Autodesk Inventor part; units mm, degrees
ref_plane "Work Plane1" through (0, -4, 9.6) normal (1, 0, 0) x (0, 0, -1)
ref_plane "YZ Plane" through (0, 0, 0) normal (1, 0, 0) x (0, 1, 0)
ref_plane "XZ Plane" through (0, 0, 0) normal (0, 1, 0) x (-1, 0, 0)
sketch "Sketch1" plane through (0, 0, 0) normal (0, 0, 1) x (1, 0, 0)
  line L0 (-4, -4) -> (4, -4)
  line L1 (4, -4) -> (4, 4)
  line L2 (4, 4) -> (-4, 4)
  line L3 (-4, 4) -> (-4, -4)
  line L4 (-4, -4) -> (4, 4) construction
  line L5 (4, -4) -> (-4, 4) construction
  circle A0 centre (0, 0) radius 2.4
  dimension "d0" = 8
  dimension "d1" = 8
  dimension "d2" = 4.8
extrude "Extrusion1" add sketch "Sketch1" along normal blind 9.6 contours L3 L2 L1 L0 | A0
extrude "Extrusion2" add sketch "Sketch1" along normal blind 11.3 contours A0
extrude "Extrusion3" cut sketch "Sketch1" along normal blind 1.7 contours A0
pattern_linear "Rectangular Pattern1" count 10 spacing 8 along (0, 1, 0) of "Extrusion1", "Extrusion2", "Extrusion3"
sketch "Sketch2" plane through (4, -4, 9.6) normal (1, 0, 0) x (0, 0, -1)
  circle A0 centre (4, 8) radius 2.4
  circle A1 centre (4, 8) radius 3.1
  line L0 (9.6, 0) -> (9.6, 80)
  line L1 (9.6, 0) -> (0, 0)
  point P0 (9.6, 4)
  dimension "d12" = 4.8
  dimension "d14" = 6.2
  dimension "d22" = 8
  dimension "d23" = 5.6
ref_plane "Work Plane1" through (0, -4, 9.6) normal (1, 0, 0) x (0, 0, -1)
extrude "Extrusion4" cut sketch "Sketch2" against normal up to next contours A0
extrude "Extrusion5" cut sketch "Sketch2" against normal blind 0.8
mirror "Mirror1" about plane through (0, -4, 9.6) normal (1, 0, 0) of "Extrusion5"
pattern_linear "Rectangular Pattern2" count 9 spacing 8 along (0, 1, 0) of "Extrusion4", "Extrusion5", "Mirror1"
equation "\"d11\" = d0"
equation "\"d21\" = d0"
properties part number "LEGO Technic Brick 1x10 with Holes"
CAD build for the part. Positions are in the model's coordinates, mm. A direction names the side the tool comes from. Round coordinates to 2 decimals unless told otherwise and drop trailing zeros. Loops run counter-clockwise (first coordinate to the right, second up) from the corner with the lowest first, then second, coordinate; pieces in that order, holes last. Notation, with made-up numbers: (4.5, -27.75) - (35.5, -27.75) arc R13 cw to (35.5, -8.75) - close; hole circle Ø9 at (45.5, -21). An arc over 180 degrees is marked (long way). Put each result on its own line as item: value.
1. Slice it at C-C on z = 6.25. Give the number of separate pieces and of enclosed holes in the cut face, and give its area (3 significant figures).
Geometry check:
separate pieces: 10
enclosed holes: 0
area: 287 mm²
2. Pin check, flat tips, straight feed: P1, Ø4, axis at x = -1, y = 16.5, coming from the -Z side; P2, Ø1, axis at x = 0, y = 47, coming from the -Z side. Stop position of each tip, or through.
Geometry check:
P1: z = 0
P2: z = 1.7
3. Wall check: line 1 (Z direction, x = 2.25, y = 47); line 2 (X direction, y = 23, z = 5.5); line 3 (Z direction, x = 3.25, y = 3.5). Give the ranges that are in metal, low to high.
Geometry check:
line 1: 0 to 9.6
line 2: -3.2 to 3.2
line 3: 0 to 2.54, 8.66 to 9.6
4. Two-plate mould, pull along Z, no slides. Class faces 6 (the cylindrical face through (-3.606, 13.187, 2.736)), 7 (the cylindrical face through (-0.31, 61.62, 10.44)), 8 (the flat face through (0, 8, 11.3)): released by +Z, released by -Z, zero draft, split by the parting line, or undercut.
Geometry check:
face 6: undercut
face 7: zero draft
face 8: released by +Z
5. Slice it at A-A on y = 28. List the corners of the cut face in (x, z).
Geometry check:
outline: (-4, 0) - (4, 0) - (4, 2.5) - (3.2, 2.5) - (3.2, 3.2) - (-3.2, 3.2) - (-3.2, 2.5) - (-4, 2.5) - close; (-4, 8.7) - (-3.2, 8.7) - (-3.2, 8) - (3.2, 8) - (3.2, 8.7) - (4, 8.7) - (4, 9.6) - (-4, 9.6) - close
6. Slice it at B-B on y = 40. List the corners of the cut face in (x, z).
Geometry check:
outline: (-4, 0) - (-2.4, 0) - (-2.4, 1.7) - (2.4, 1.7) - (2.4, 0) - (4, 0) - (4, 9.6) - (2.4, 9.6) - (2.4, 11.3) - (-2.4, 11.3) - (-2.4, 9.6) - (-4, 9.6) - close
7. 3-axis set-ups, long thin cutter, end or side, ignore diameter. For faces 1 (the cylindrical face through (1.29, 13.976, 10.438)), 2 (the cylindrical face through (0.045, 62.024, 4.31)), 3 (the cylindrical face through (-3.606, 64.926, 6.004)), 4 (the flat face through (0, 8, 1.7)), 5 (the flat face through (3.2, 50, 4)): which of +Z, -Z, +X, -X, +Y, -Y reach the whole face in a straight line?
Geometry check:
face 1: +Z
face 2: +X, -X
face 3: -X
face 4: -Z
face 5: +X
